Read the model definition and answer for the solid it produces. Units are mm, in the model's axes. Face numbers are marked on the shaded views. A direction names the side the tool comes from. Round coordinates to 2 decimals unless told otherwise and drop trailing zeros. Order: outer loops, then holes, each group sorted by start corner. A loop starts at its lowest first (then second) coordinate and runs counter-clockwise, first axis right, second up.
Autodesk Inventor part; units mm, degrees
ref_plane "YZ Plane" through (0, 0, 0) normal (1, 0, 0) x (0, 1, 0)
ref_plane "XZ Plane" through (0, 0, 0) normal (0, 1, 0) x (-1, 0, 0)
ref_plane "XY Plane" through (0, 0, 0) normal (0, 0, 1) x (1, 0, 0)
sketch "Эскиз1" plane through (0, 0, 0) normal (0, 0, 1) x (1, 0, 0)
  line L0 (0, 0) -> (78, 0)
  line L1 (78, 0) -> (78, 24)
  line L2 (78, 24) -> (120, 24)
  line L3 (120, 24) -> (120, 49)
  line L4 (120, 49) -> (0, 49)
  line L5 (65.5, 20.9431) -> (0, 20.9431)
  line L6 (0, 49) -> (0, 20.9431)
  line L7 (65.5, 20.9431) -> (65.5, 0)
  line L8 (65.5, 0) -> (73.5, 0)
  line L9 (73.5, 0) -> (78, 13.3185)
  line L10 (78, 14.7395) -> (74, 14.7395)
  line L11 (74, 14.7395) -> (74, 19.7395)
  line L12 (74, 19.7395) -> (78, 19.7395)
  dimension "d0" = 78
  dimension "d1" = 24
  dimension "d2" = 42
  dimension "d3" = 25
  dimension "d18" = 65.5
  dimension "d19" = 8
  dimension "d21" = 4
  dimension "d22" = 5
revolve "Вращение1" add sketch "Эскиз1" angle 360 about axis through (0, 49, 0) along (0, -1, 0) contours L7 L5 L6 L4 L3 L2 L1 L12 L11 L10 L9 L0
sketch "Эскиз2" plane through (0, 49, 0) normal (0, 1, 0) x (1, 0, 0)
  circle A0 centre (0, 0) radius 120
  line L0 (120, 0) -> (99.5, 0)
  point P0 (0, 0)
  dimension "d7" = 20.5
hole "Отверстие1" at (99.5, 49, 0) direction (0, -1, 0) diameter 22 end through all
pattern_circular "Круговой массив1" count 10 over 360 about axis through (0, 10.4715, 0) along (0, -1, 0) of "Отверстие1"
fillet "Сопряжение1" radius 10 1 edges at (-65.5, 20.9431, 0)
properties part number "Крышка стакана" material "Чугун, серый"
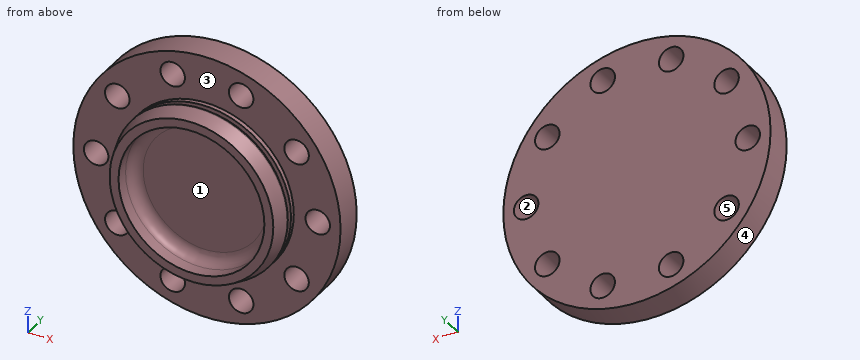
Q1. Straight lines are drawn through the part: probe 1 along Y at (x, z) = (-105.5, -29); probe 2 along Z at (x, y) = (22, 27.5); probe 3 along X at (y, z) = (38.5, -89.5). For each, find the intervals that lie inside material, in ascending order.
Outcome:
probe 1: y = 24 to 49
probe 2: z = -117.97 to -101.3, -87.96 to 87.96, 101.3 to 117.97
probe 3: x = -79.94 to -40.48, -21.02 to 21.02, 40.48 to 79.94
Q2. For a pull along Z with two mould halves and no side action, classify the marked faces 3, 4 and 5 as released by +Z, released by -Z, zero draft, split by the parting line, or undercut.
Outcome:
face 3: zero draft
face 4: split by the parting line
face 5: undercut
Q3. For the marked faces 1 and 2, determine the directions among +Z, -Z, +X, -X, +Y, -Y from which every point of the face is accessible in a straight line to the end or side of a thin tool.
Outcome:
face 1: -Y
face 2: +Y, -Y
Q4. Flat-ended cylindrical pins translate along their axes: pin 1 (3 mm diameter, centred on y = 39, z = 56, fed in from +X); pin 2 (2 mm diameter, centred on y = 40, z = -62, fed in from +X); pin 3 (5 mm diameter, centred on x = -49.5, z = -6.5, fed in from -Y). Find the tip coordinate at first contact, or state that the pin passes through.
Outcome:
pin 1: stops at x = 106.91
pin 2: stops at x = 103.34
pin 3: stops at y = 20.94
Q5. A cutting plane is placed at B-B, the plane x = 99.5. Give the vertices of the cut face in (y, z), plus the area to 3 significant figures.
Outcome:
outline: (24, -67.08) - (49, -67.08) - (49, -11) - (24, -11) - close; (24, 11) - (49, 11) - (49, 67.08) - (24, 67.08) - close
area: 2,800 mm2
Q6. A cutting plane is placed at C-C, the plane x = 0. Give the vertices of the cut face in (y, z), plus the area to 3 significant figures.
Outcome:
outline: (0, -73.5) - (13.32, -78) - (14.74, -78) - (14.74, -74) - (19.74, -74) - (19.74, -78) - (24, -78) - (24, -120) - (49, -120) - (49, 120) - (24, 120) - (24, 78) - (19.74, 78) - (19.74, 74) - (14.74, 74) - (14.74, 78) - (13.32, 78) - (0, 73.5) - (0, 65.5) - (10.94, 65.5) arc R10 cw to (20.94, 55.5) - (20.94, -55.5) arc R10 cw to (10.94, -65.5) - (0, -65.5) - close
area: 6,940 mm2
Q7. A cutting plane is placed at A-A, the plane z = 0. Give the number of separate pieces and of enclosed holes in the cut face, plus the area to 3 significant figures.
Outcome:
separate pieces: 3
enclosed holes: 0
area: 5,840 mm2
